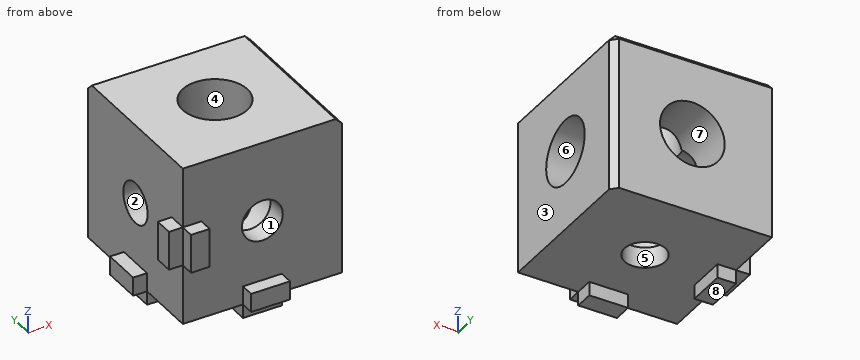
from build123d import *

# Parameters (mm, degrees)
SKETCH1_W           = 25.4
SKETCH1_H           = 25.4
BOSS_EXTRUDE1_DEPTH = 25.4
SKETCH6_W           = 2.96999914
SKETCH6_H           = 6.19999776
BOSS_EXTRUDE2_DEPTH = 2.20999812
BOSS_EXTRUDE3_REACH = 42.371
SKETCH7_W           = 6.19999776
SKETCH7_H           = 2.96999914
SKETCH8_W           = 6.19999776
SKETCH8_H           = 2.96999914
BOSS_EXTRUDE4_DEPTH = 2.20999812
BOSS_EXTRUDE5_REACH = 42.371
SKETCH9_W           = 6.19999776
SKETCH9_H           = 2.96999914
SKETCH10_W          = 2.96999914
SKETCH10_H          = 6.19999776
BOSS_EXTRUDE6_DEPTH = 2.20999812
BOSS_EXTRUDE7_REACH = 42.371
SKETCH11_W          = 2.96999914
SKETCH11_H          = 6.19999776
HOLE3_REACH         = 42.371
HOLE3_BORE_R        = 5.15999984
HOLE4_D             = 6.51999712
HOLE4_CBORE_D       = 10.31999968
HOLE4_CBORE_DEPTH   = 22.09999898
CHAMFER1_SIZE       = 1.016


with BuildPart() as part:
    # Sketch1 → Boss-Extrude1 (new body)
    with BuildSketch(Plane(origin=(0, 25.4, 0), x_dir=(1, 0, 0), z_dir=(0, 1, 0))):
        Rectangle(SKETCH1_W, SKETCH1_H)
    extrude(amount=-BOSS_EXTRUDE1_DEPTH)

    # Sketch2 → Hole1 (revolve, cut)
    with BuildSketch(Plane(origin=(0, 0, 0), x_dir=(0, 0, -1), z_dir=(1, 0, 0))):
        Polygon((0, 0), (0, 25.4), (5.15999984, 25.4), (5.15999984, 3.30000102), (3.25999856, 3.30000102), (3.25999856, 0), align=None)
    revolve(axis=Axis((0, 110, 0), (0, -1, 0)), mode=Mode.SUBTRACT)

    # Sketch4 → Hole2 (revolve, cut)
    with BuildSketch(Plane(origin=(0, 12.7, -12.7), x_dir=(0, 1, 0), z_dir=(1, 0, 0))):
        Polygon((0, 0), (0, 12.7), (5.15999984, 12.7), (5.15999984, 3.30000102), (3.25999856, 3.30000102), (3.25999856, 0), align=None)
    revolve(axis=Axis((0, 12.7, 97.3), (0, 0, -1)), mode=Mode.SUBTRACT)

    # Sketch6 → Boss-Extrude2 (add)
    with BuildSketch(Plane(origin=(0, 0, -12.7), x_dir=(-1, 0, 0), z_dir=(0, 0, -1))):
        with Locations((11.21500043, 12.7)):
            Rectangle(SKETCH6_W, SKETCH6_H)
    extrude(amount=BOSS_EXTRUDE2_DEPTH)

    # Sketch7 → Boss-Extrude3 (add, up to next)
    with BuildSketch(Plane(origin=(-14.90999812, 0, 0), x_dir=(0, -1, 0), z_dir=(-1, 0, 0)), mode=Mode.PRIVATE) as boss_extrude3_sk1:
        with Locations((-12.7, -11.21500043)):
            Rectangle(SKETCH7_W, SKETCH7_H)
    boss_extrude3_tool1 = extrude(boss_extrude3_sk1.sketch, amount=-BOSS_EXTRUDE3_REACH, mode=Mode.PRIVATE) - part.part
    add(boss_extrude3_tool1.solids().sort_by_distance((-14.909998, 12.7, -11.215))[0])

    # Sketch8 → Boss-Extrude4 (add)
    with BuildSketch(Plane.XZ):
        with Locations((0, -11.21500043)):
            Rectangle(SKETCH8_W, SKETCH8_H)
    extrude(amount=BOSS_EXTRUDE4_DEPTH)

    # Sketch9 → Boss-Extrude5 (add, up to next)
    with BuildSketch(Plane(origin=(0, 0, -14.90999812), x_dir=(-1, 0, 0), z_dir=(0, 0, -1)), mode=Mode.PRIVATE) as boss_extrude5_sk1:
        with Locations((0, 1.48499957)):
            Rectangle(SKETCH9_W, SKETCH9_H)
    boss_extrude5_tool1 = extrude(boss_extrude5_sk1.sketch, amount=-BOSS_EXTRUDE5_REACH, mode=Mode.PRIVATE) - part.part
    add(boss_extrude5_tool1.solids().sort_by_distance((0, 1.485, -14.909998))[0])

    # Sketch10 → Boss-Extrude6 (add)
    with BuildSketch(Plane.XZ):
        with Locations((-11.21500043, 0)):
            Rectangle(SKETCH10_W, SKETCH10_H)
    extrude(amount=BOSS_EXTRUDE6_DEPTH)

    # Sketch11 → Boss-Extrude7 (add, up to next)
    with BuildSketch(Plane(origin=(-14.90999812, 0, 0), x_dir=(0, -1, 0), z_dir=(-1, 0, 0)), mode=Mode.PRIVATE) as boss_extrude7_sk1:
        with Locations((-1.48499957, 0)):
            Rectangle(SKETCH11_W, SKETCH11_H)
    boss_extrude7_tool1 = extrude(boss_extrude7_sk1.sketch, amount=-BOSS_EXTRUDE7_REACH, mode=Mode.PRIVATE) - part.part
    add(boss_extrude7_tool1.solids().sort_by_distance((-14.909998, 1.485, 0))[0])

    # Hole3 bore → Hole3 (cut, up to next)
    with BuildSketch(Plane.XY.offset(12.7), mode=Mode.PRIVATE) as hole3_sk1:
        with Locations((0, 12.7)):
            Circle(HOLE3_BORE_R)
    hole3_tool1 = extrude(hole3_sk1.sketch, amount=-HOLE3_REACH, mode=Mode.PRIVATE) & part.part
    add(hole3_tool1.solids().sort_by_distance((0, 12.7, 12.7))[0], mode=Mode.SUBTRACT)

    # Hole4 (through all)
    with Locations(Plane(origin=(12.7, 0, 0), x_dir=(0, 0, -1), z_dir=(1, 0, 0))):
        with Locations((0, 12.7)):
            CounterBoreHole(HOLE4_D / 2, HOLE4_CBORE_D / 2, HOLE4_CBORE_DEPTH)

    # Chamfer1
    chamfer1_edges = [part.edges().sort_by_distance(p)[0] for p in [
        (12.7, 25.4, 0),
        (0, 25.4, 12.7),
        (12.7, 12.7, 12.7),
    ]]
    chamfer(chamfer1_edges, length=CHAMFER1_SIZE)


solid = part.part
Verification items for the finished model (mm, model axes). Face numbers are marked on the shaded views. A direction names the side the tool comes from. Coordinates: 2 decimals unless noted, no trailing zeros. Order: outer loops, then holes, each group sorted by start corner. A loop starts at its lowest first (then second) coordinate and runs counter-clockwise, first axis right, second up.
Item 1: Access from +Z, -Z, +X, -X, +Y, -Y to the whole of each face (thin tool, end or side, straight path). Record for the marked faces 4, 5, 6, 7 and 8.
Filled in:
face 4: +Z
face 5: +Z, -Z
face 6: +X
face 7: +Y
face 8: -Z, +X, -X, +Y, -Y
Item 2: Material ranges on L1, parallel to Y at x = 0, z = 8.25; L2, parallel to Z at x = 0, y = 6.65, recorded low to high.
Filled in:
L1: y = 0 to 7.54, 17.86 to 25.4
L2: z = -12.7 to -5.16, 5.16 to 12.7
Item 3: Section check C-C, the plane x = -12.25. Enter the section's corners in (y, z).
Filled in:
outline: (-2.21, -3.1) - (0, -3.1) - (0, -12.7) - (9.6, -12.7) - (9.6, -14.91) - (15.8, -14.91) - (15.8, -12.7) - (25.4, -12.7) - (25.4, 11.68) - (24.38, 12.7) - (0, 12.7) - (0, 3.1) - (-2.21, 3.1) - close; hole circle Ø6.52 at (12.7, 0)
Item 4: Section check D-D, the plane y = 6. Enter the section's corners in (x, z), then the cut area to 3 significant figures.
Filled in:
outline: (-12.7, -12.7) - (12.7, -12.7) - (12.7, 11.68) - (11.68, 12.7) - (-12.7, 12.7) - close; hole circle Ø10.32 at (0, 0)
area: 561 mm2
Item 5: Section check A-A, the plane z = 0. Give the number of separate pieces and of enclosed holes in the cut face, then the cut area to 3 significant figures.
Filled in:
separate pieces: 4
enclosed holes: 0
area: 265 mm2
Item 6: Release check for a two-part mould opening along X. For the marked faces 1, 2 and 3 record: +X half, -X half, draft (parallel to the pull), parting line (faces both ways), or undercut.
Filled in:
face 1: undercut
face 2: draft
face 3: +X half
Item 7: Depth check by flat-ended pin: pin 1 (12 mm diameter, centred on x = 0, y = 12.7, fed in from -Z); pin 2 (2.5 mm diameter, centred on y = -1.5, z = -0.5, fed in from -X); pin 3 (3 mm diameter, centred on x = 2.5, z = -1.5, fed in from +Y); pin 4 (6 mm diameter, centred on x = 0, y = 12.7, fed in from +Z). Enter the tip coordinate at first touch or a pass-through.
Filled in:
pin 1: stops at z = -12.7
pin 2: stops at x = -12.7
pin 3: stops at y = 3.3
pin 4: passes through
